Input: part model. Units: mm. Frame: model coordinates. Face numbers are marked on the shaded views. A direction names the side the tool comes from. Round coordinates to 2 decimals unless told otherwise and drop trailing zeros. Write each loop counter-clockwise with the first axis right and the second up, starting at its lowest first coordinate (ties: lowest second). Pieces come first, ordered by that corner, then holes. Notation, with made-up numbers: (42.25, -37) - (78.25, -37) arc R31 ccw to (78.25, 2) - close; hole circle Ø9 at (34.25, -35). An arc over 180 degrees is marked (long way). Use one line per item in the form item = value.
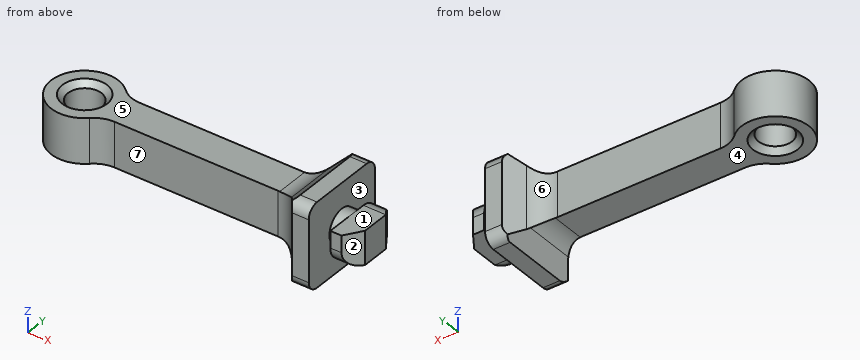
```python
from build123d import *

# Parameters (mm, degrees)
F0_R      = 3
F1_DEPTH  = 15
F2_R      = 3
F3_DEPTH  = 2
F5_DEPTH  = 4
F7_DEPTH  = 25
F9_DEPTH  = 25
F11_DEPTH = 25
F12_SIZE  = 1
F13_SIZE  = 1
F14_R     = 2
F15_R     = 2
F16_R     = 3


# Not quite as in the source:
# - a feature names something its author has since deleted; it is built from what else it names


with BuildPart() as f1:
    # F0 (on Top) → F1 (new body)
    with BuildSketch(Plane.XY):
        with BuildLine():
            ThreePointArc((-38.3954955959, 25.79224433), (-40.2418679606, 26.1456424436), (-41.8272385211, 27.1558806937))
            ThreePointArc((-41.8272385211, 27.1558806937), (-51.9453300312, 22.79224433), (-41.8272385211, 18.4286079664))
            ThreePointArc((-41.8272385211, 18.4286079664), (-40.2418679606, 19.4388462165), (-38.3954955959, 19.79224433))
            Line((-38.3954955959, 19.79224433), (-9.2304363188, 19.79224433))
            ThreePointArc((-9.2304363188, 19.79224433), (-6.9849852462, 19.2596764203), (-5.2178762474, 17.7754241224))
            Line((-5.2178762474, 17.7754241224), (-3, 14.79224433))
            Line((-3, 14.79224433), (0, 14.79224433))
            Line((0, 14.79224433), (0, 19.79224433))
            Line((0, 19.79224433), (0, 25.79224433))
            Line((0, 25.79224433), (0, 30.79224433))
            Line((0, 30.79224433), (-3, 30.79224433))
            Line((-3, 30.79224433), (-5.2178762474, 27.8090645377))
            ThreePointArc((-5.2178762474, 27.8090645377), (-6.9849852462, 26.3248122398), (-9.2304363188, 25.79224433))
            Line((-9.2304363188, 25.79224433), (-38.3954955959, 25.79224433))
        make_face()
        with Locations((-45.9453300312, 22.79224433)):
            Circle(F0_R, mode=Mode.SUBTRACT)
    extrude(amount=F1_DEPTH)

    # F2 (on face) → F3 (join)
    with BuildSketch(Plane.YZ):
        with Locations((22.79224433, 7.5)):
            Circle(F2_R)
    extrude(amount=F3_DEPTH)

    # F4 (on face) → F5 (join)
    with BuildSketch(Plane.YZ.offset(2)):
        Polygon((17.29224433, 4.5), (26.29224433, 4.5), (28.29224433, 4.5), (28.29224433, 6), (28.29224433, 10.5), (19.29224433, 10.5), (17.29224433, 10.5), (17.29224433, 9), align=None)
    extrude(amount=F5_DEPTH)

    # F6 (on face) → F7 (cut)
    with BuildSketch(Plane(origin=(0, 0, 4.5), x_dir=(1, 0, 0), z_dir=(0, 0, -1))):
        Polygon((6, -17.29224433), (4, -17.29224433), (6, -20.29224433), align=None)
    extrude(amount=-F7_DEPTH, mode=Mode.SUBTRACT)

    # F8 (on face) → F9 (cut)
    with BuildSketch(Plane.XY.offset(10.5)):
        Polygon((6, 28.29224433), (4, 28.29224433), (6, 25.29224433), align=None)
    extrude(amount=-F9_DEPTH, mode=Mode.SUBTRACT)

    # F10 (on face) → F11 (cut)
    with BuildSketch(Plane.XZ.offset(-14.79224433)):
        with BuildLine():
            Line((-52.1873838902, 19.9649333954), (-52.1873838902, 11.5))
            Line((-52.1873838902, 11.5), (-8.8786755805, 11.5))
            ThreePointArc((-8.8786755805, 11.5), (-7.1200422145, 11.8194862799), (-5.5861525412, 12.7371165265))
            Line((-5.5861525412, 12.7371165265), (-3, 15))
            Line((-3, 15), (-3, 19.9649333954))
            Line((-3, 19.9649333954), (-52.1873838902, 19.9649333954))
        make_face()
        with BuildLine():
            Line((-2.2940631025, -5.0414614379), (-3, 0))
            Line((-3, 0), (-5.5861525412, 2.2628834735))
            ThreePointArc((-5.5861525412, 2.2628834735), (-7.1200422145, 3.1805137201), (-8.8786755805, 3.5))
            Line((-8.8786755805, 3.5), (-52.6222039647, 3.5))
            Line((-52.6222039647, 3.5), (-52.6222039647, -5.0414614379))
            Line((-52.6222039647, -5.0414614379), (-2.2940631025, -5.0414614379))
        make_face()
    extrude(amount=-F11_DEPTH, mode=Mode.SUBTRACT)

    # F12
    f12_edges = [f1.edges().sort_by_distance(p)[0] for p in [
        (-48.94533, 22.792244, 11.5),
    ]]
    chamfer(f12_edges, length=F12_SIZE)

    # F13
    f13_edges = [f1.edges().sort_by_distance(p)[0] for p in [
        (-48.94533, 22.792244, 3.5),
    ]]
    chamfer(f13_edges, length=F13_SIZE)

    # F14
    f14_edges = [f1.edges().sort_by_distance(p)[0] for p in [
        (-1.5, 14.792244, 15),
    ]]
    fillet(f14_edges, radius=F14_R)

    # F15
    f15_edges = [f1.edges().sort_by_distance(p)[0] for p in [
        (-1.5, 30.792244, 15),
        (-1.5, 30.792244, 0),
        (-1.5, 14.792244, 0),
    ]]
    fillet(f15_edges, radius=F15_R)

    # F16
    f16_edges = [f1.edges().sort_by_distance(p)[0] for p in [
        (3, 17.292244, 4.5),
        (3, 28.292244, 10.5),
    ]]
    fillet(f16_edges, radius=F16_R)


solid = f1.part
```
(1) Material intervals for L1, parallel to X at y = 25.5, z = 6; L2, parallel to X at y = 27.25, z = 8.5; L3, parallel to Y at x = -15, z = 6, sorted ascending.
Derived:
L1 = -51.3 to -47.24, -44.65 to 0, 2 to 5.86
L2 = -49.96 to -41.93, -5.7 to 0, 2 to 4.69
L3 = 19.79 to 25.79
(2) Cut plane B-B on z = 14. Output: boundary loops of the cut face in (x, y).
Derived:
outline = (-4.14, 16.33) - (-3.2, 15.06) - (0, 15.06) - (0, 30.52) - (-3.2, 30.52) - (-4.14, 29.26) - close
(3) Cut plane C-C on x = -23.5. Output: boundary loops of the cut face in (y, z), then the cut area to 3 significant figures.
Derived:
outline = (19.79, 3.5) - (25.79, 3.5) - (25.79, 11.5) - (19.79, 11.5) - close
area = 48.0 mm^2
(4) First-contact query: pin 1 Ø9.5 at (x, y) = (-30, 22) entering from +Z; pin 2 Ø5 at (x, z) = (-11.5, 6) entering from -Y; pin 3 Ø6 at (x, y) = (-27, 25) entering from -Z; pin 4 Ø6 at (y, z) = (24.5, 1.5) entering from -X. Flat tips, straight axial feed; report the tip coordinate or a pass-through.
Derived:
pin_1 = 11.5
pin_2 = 19.79
pin_3 = 3.5
pin_4 = -51.95
(5) Cut plane A-A on z = 8.25. Output: boundary loops of the cut face in (x, y), then the cut area to 3 significant figures.
Derived:
outline = (-41.83, 18.43) arc R5 cw to (-38.4, 19.79) - (-9.23, 19.79) arc R5 cw to (-5.22, 17.78) - (-3, 14.79) - (0, 14.79) - (0, 19.89) - (2, 19.89) - (2, 17.29) - (4, 17.29) - (6, 20.29) - (6, 25.29) - (4.06, 28.2) - (2, 28.2) - (2, 25.7) - (0, 25.7) - (0, 30.79) - (-3, 30.79) - (-5.22, 27.81) arc R5 cw to (-9.23, 25.79) - (-38.4, 25.79) arc R5 cw to (-41.83, 27.16) arc R6 ccw (long way) to start; hole circle Ø6 at (-45.95, 22.79)
area = 427 mm^2
(6) Access query for the marked faces 4, 5, 6 and 7. Directions: +Z, -Z, +X, -X, +Y, -Y. A direction counts if a zero-diameter tool reaches every point of the face in a straight line with its end or side. Return the directions, or none.
Derived:
face_4 = -Z, -X, +Y, -Y
face_5 = +Z, -X, +Y, -Y
face_6 = +Z, -Z, +Y
face_7 = +Z, -Z, -Y
(7) Draft query along X for the marked faces 1, 2 and 3. Return one class per face: released by +X, released by -X, zero draft, split by the parting line, or undercut.
Derived:
face_1 = zero draft
face_2 = released by +X
face_3 = undercut
